```python
from build123d import *

# Parameters (mm, degrees)
SKETCH_1_R          = 13.5
EXTRUDE_1_DEPTH     = 4
SKETCH_2_R          = 6
EXTRUDE_2_DEPTH     = 11
SKETCH_3_R          = 4
CUT_EXTRUDE_1_DEPTH = 25.279621084
SKETCH_4_R          = 1.75
CUT_EXTRUDE_2_DEPTH = 25.279621084
SKETCH_5_R          = 3
CUT_EXTRUDE_3_DEPTH = 2.2
CHAMFER_1_SIZE      = 0.2


with BuildPart() as part:
    # 草图1 → 凸台-拉伸1 (new body)
    with BuildSketch(Plane(origin=(0, 0, 0), x_dir=(1, 0, 0), z_dir=(0, 1, 0))):
        with Locations(Location((0, 0, 0), (0, 0, 270))):
            Circle(SKETCH_1_R)
    extrude(amount=EXTRUDE_1_DEPTH)

    # 草图2 → 凸台-拉伸2 (add)
    with BuildSketch(Plane(origin=(0, 4, 0), x_dir=(1, 0, 0), z_dir=(0, 1, 0))):
        with Locations(Location((0, 0, 0), (0, 0, 270))):
            Circle(SKETCH_2_R)
    extrude(amount=EXTRUDE_2_DEPTH)

    # 草图3 → 切除-拉伸1 (cut, through all)
    with BuildSketch(Plane(origin=(0, 0, 0), x_dir=(-1, 0, 0), z_dir=(0, -1, 0))):
        with Locations(Location((0, 0, 0), (0, 0, 90))):
            Circle(SKETCH_3_R)
    extrude(amount=-CUT_EXTRUDE_1_DEPTH, mode=Mode.SUBTRACT)

    # 草图4 → 切除-拉伸2 (cut, through all)
    with BuildSketch(Plane.XZ):
        with Locations(Location((0, 9.5, 0), (0, 0, 270))):
            Circle(SKETCH_4_R)
        with Locations(Location((0, -9.5, 0), (0, 0, 270))):
            Circle(SKETCH_4_R)
    extrude(amount=-CUT_EXTRUDE_2_DEPTH, mode=Mode.SUBTRACT)

    # 草图5 → 切除-拉伸3 (cut)
    with BuildSketch(Plane(origin=(0, 0, 0), x_dir=(-1, 0, 0), z_dir=(0, -1, 0))):
        with Locations(Location((0, -9.5, 0), (0, 0, 90))):
            Circle(SKETCH_5_R)
        with Locations(Location((0, 9.5, 0), (0, 0, 90))):
            Circle(SKETCH_5_R)
    extrude(amount=-CUT_EXTRUDE_3_DEPTH, mode=Mode.SUBTRACT)

    # 倒角1
    chamfer_1_edges = [part.edges().sort_by_distance(p)[0] for p in [
        (0, 15, 4),
        (0, 0, -13.5),
        (0, 4, -13.5),
        (0, 15, -6),
    ]]
    chamfer(chamfer_1_edges, length=CHAMFER_1_SIZE)


solid = part.part
```
Geometry check sheet. Reference: the model listing, model coordinates, mm. A direction names the side the tool comes from. Give positions to 0.01 mm unless a question says otherwise; leave off trailing zeros. Order: outer loops, then holes, each group sorted by start corner. A loop starts at its lowest first (then second) coordinate and runs counter-clockwise, first axis right, second up. Notation, with made-up numbers: (65.25, 1) - (117.25, 1) arc R14 ccw to (117.25, 18) - close; hole circle Ø7 at (80.5, -24). An arc over 180 degrees is marked (long way). Write item = value, one per line. Start each with the question number.
1) Section check A-A (z = 0). Enter the section's corners in (x, y), then the cut area to 3 significant figures.
2) Scan lines: L1, parallel to Y at x = -5.25, z = -6.75; L2, parallel to X at y = 3.3, z = 9.5; L3, parallel to Z at x = -0.5, y = 12.75. Record each from-to range of solid material in increasing order.
3) Section check B-B (x = 0). Count the separate pieces of the cut face and the enclosed holes in it, then the cut area to 3 significant figures.
4) Section check C-C (y = 6.5). Enter the section's corners in (x, z), then the cut area to 3 significant figures.
5) Gauge pin test, flat ends, axial feed: pin 1 Ø1 at (x, y) = (-6, 2.5) entering from +Z; pin 2 Ø1.5 at (x, y) = (-2, 2) entering from +Z; pin 3 Ø10 at (x, z) = (1, -0.5) entering from +Y; pin 4 Ø6 at (x, y) = (-7, 9) entering from +Z. Record the tip position at first contact, or that the pin passes through.
6) Draft check along X on faces 4 (the cylindrical face through (1.802, 9.324, 5.723)), 5 (the flat face through (2, 15, 4)), 6 (the cylindrical face through (-1.15, 1.08, -12.27)), 7 (the cylindrical face through (-0.67, 3.087, 7.883)). Enter one of: released by +X, released by -X, zero draft, split by the parting line, or undercut.
7) Access from +Z, -Z, +X, -X, +Y, -Y to the whole of each face (thin tool, end or side, straight path). Record for faces 1 (the flat face through (3, 0, 3)), 2 (the flat face through (0, 2.2, 7.5)), 3 (the flat face through (-3, 4, 6)).
Geometry check:
q1.outline = (-13.5, 0.2) - (-13.3, 0) - (-4, 0) - (-4, 14.8) - (-4.2, 15) - (-5.8, 15) - (-6, 14.8) - (-6, 4) - (-13.3, 4) - (-13.5, 3.8) - close; (4, 0) - (13.3, 0) - (13.5, 0.2) - (13.5, 3.8) - (13.3, 4) - (6, 4) - (6, 14.8) - (5.8, 15) - (4.2, 15) - (4, 14.8) - close
q1.area = 120 mm2
q2.L1 = 0 to 4
q2.L2 = -9.59 to -1.75, 1.75 to 9.59
q2.L3 = -5.98 to -3.97, 3.97 to 5.98
q3.separate_pieces = 4
q3.enclosed_holes = 0
q3.area = 80.8 mm2
q4.outline = circle Ø12 at (0, 0); hole circle Ø8 at (0, 0)
q4.area = 62.8 mm2
q5.pin_1 = 12.33
q5.pin_2 = 13.44
q5.pin_3 = 15
q5.pin_4 = 4.47
q6.face_4 = split by the parting line
q6.face_5 = zero draft
q6.face_6 = undercut
q6.face_7 = undercut
q7.face_1 = +Z, -Z, +X, -X, -Y
q7.face_2 = -Y
q7.face_3 = +Y
